Drawing for the job (mm, zero at the part's lowest x, y, z). A direction names the side the tool comes from. Round coordinates to 2 decimals unless told otherwise and drop trailing zeros. Loops run counter-clockwise (first coordinate to the right, second up) from the corner with the lowest first, then second, coordinate; pieces in that order, holes last. Notation, with made-up numbers: (-23.5, 67) -> (27.5, 67) arc R6 cw to (27.5, 77) -> close; hole circle Ø5 at (-16.5, 1.25). An arc over 180 degrees is marked (long way). Put each result on its own line as item: value. Start each with the question number.
Item 1: Cut at B-B, the plane z = 200.5. List the corners of the cut face in (x, y), plus the area to 3 significant figures.
Item 2: Cut at C-C, the plane z = 41. List the corners of the cut face in (x, y).
Item 3: Flat gauge pins, fed straight in: pin 1 Ø10 at (y, z) = (176, 27.5) entering from +X; pin 2 Ø4 at (x, z) = (102, 144) entering from +Y (3 decimals); pin 3 Ø3 at (x, y) = (184.5, 79) entering from +Z. Where does each tip first touch, or does it go through?
Item 4: Drill centre lines: probe 1 along Y at (x, z) = (100.5, 46); probe 2 along Z at (x, y) = (67.5, 32.5); probe 3 along Y at (x, z) = (175, 171). Where is each one in solid material? Low to high. Write a range as [from, to].
Item 5: Cut at A-A, the plane x = 125. List the corners of the cut face in (y, z).
Item 6: Tool access for the marked faces 1 and 2: list every direction of +Z, -Z, +X, -X, +Y, -Y with a clear straight run to the whole face (end or side of a thin tool).
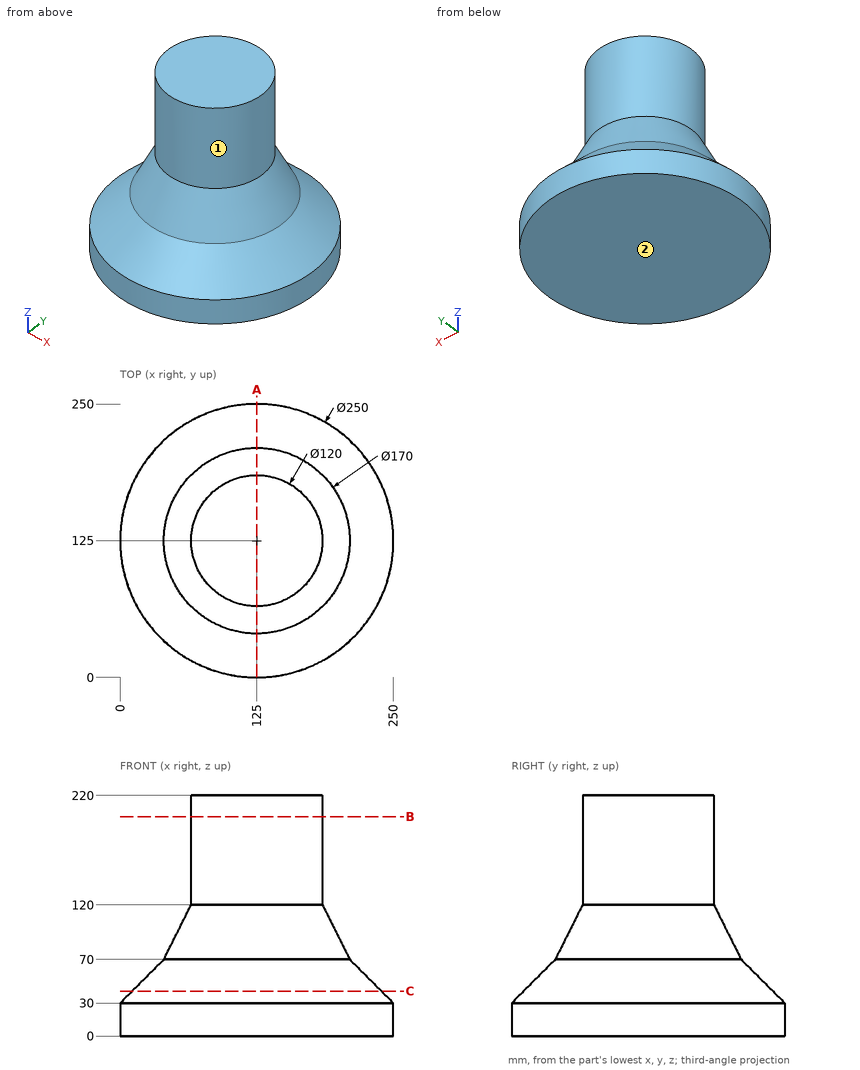
Reply:
1. outline: circle Ø120 at (125, 125)
1. area: 11,300 mm^2
2. outline: circle Ø228 at (125, 125)
3. pin 1: stops at x = 241.23
3. pin 2: stops at y = 181.205
3. pin 3: stops at z = 92.58
4. probe 1: y = [18.79, 231.21]
4. probe 2: z = [0, 46.08]
4. probe 3: y = [91.83, 158.17]
5. outline: (0, 0) -> (250, 0) -> (250, 30) -> (210, 70) -> (185, 120) -> (185, 220) -> (65, 220) -> (65, 120) -> (40, 70) -> (0, 30) -> close
6. face 1: +Z
6. face 2: -Z, +X, -X, +Y, -Y
